Could you check a few things on this model? Use its own coordinates, in mm. A direction names the side the tool comes from. Round coordinates to 2 decimals unless told otherwise and drop trailing zeros. Write each loop counter-clockwise with the first axis right and the second up, starting at its lowest first coordinate (ties: lowest second). Pieces come first, ordered by that corner, then holes. Notation, with made-up numbers: M 35,42.25 L 78,42.25 A21 ccw 78,62.25 Z; hole C -29.75,57 d8. An arc over 180 degrees is marked long. One line per item, written item: value. Start each with the question number.
(1) Which directions (+Z, -Z, +X, -X, +Y, -Y) give clear straight access to the entire face, cutting with the end or side of a thin tool? Please do faces 4 (the face through (10.175, -5, 10)), 5 (the face through (-0.222, 6.984, 21.479)), 6 (the face through (3.32, 20.29, 17.54)), 7 (the face through (-9.906, -5, 10)).
(2) If I drill on L1, parallel to X at y = -4.5, z = 14.5; L2, parallel to Z at x = -0.5, y = 13; L3, parallel to Z at x = -4, y = 18.5, over which ranges is the centre line in solid material (lowest first)?
(3) I want a section at A-A on z = 1.5. Please give me the cut outline in (x, y), and give its area (3 significant figures).
(4) Thinking about a two-plate mould opening in Y: for faces 1 (the face through (14.93, 20.13, 9.86)), 2 (the face through (1.735, -1.567, 17.535)), 3 (the face through (15.17, 5.05, 9.86)), which applies, released by +Y, released by -Y, zero draft, split by the parting line, or undercut?
(5) I want a section at B-B on y = -3. Please give me the cut outline in (x, z), and give its area (3 significant figures).
(6) I want a section at C-C on x = -7. Please give me the cut outline in (y, z).
(7) I want a section at D-D on y = 22.5. Please give me the cut outline in (x, z), and give its area (3 significant figures).
(8) I'm going to push flat-ended pins straight in: pin 1 Ø6 at (x, y) = (-1, -1) entering from +Z; pin 2 Ø8 at (y, z) = (-5, 8) entering from +X; pin 3 Ø3 at (x, z) = (-14, 14) entering from +Y. Where does each tip first touch, or does it pass through?
```python
from build123d import *

# Parameters (mm, degrees)
PAD_DEPTH       = 20
POCKET_DEPTH    = 5
POCKET001_DEPTH = 5
PAD001_DEPTH    = 3


with BuildPart() as part:
    # Sketch → Pad (new body)
    with BuildSketch(Plane.XY):
        Polygon((-10.101072, 30.032787), (9.979783, 30.032787), (20.020205, 9.951933), (10.174738, 0), (10.174738, -9.836479), (-9.906112, -9.836479), (-9.906112, 0), (-20.141495, 9.854452), align=None)
    extrude(amount=PAD_DEPTH)

    # Sketch001 (on Face10 of Pad) → Pocket (cut)
    with BuildSketch(Plane.XY.offset(20)):
        Polygon((-6.373003, -1.744858), (-6.373003, -9.245775), (-5.063322, -9.126713), (-4.825196, -1.625796), align=None)
        Polygon((-3.158328, -1.506734), (-3.158328, -9.483899), (-1.253332, -9.364837), (-1.015209, -1.506734), align=None)
        Polygon((0.889791, -1.506734), (0.770723, -8.888589), (2.437592, -8.888589), (2.556656, -1.625796), align=None)
        Polygon((4.342592, -1.268609), (4.104469, -8.769526), (6.128524, -8.769526), (6.485711, -1.506734), align=None)
    extrude(amount=-POCKET_DEPTH, mode=Mode.SUBTRACT)

    # Sketch002 (on Face5 of Pocket) → Pocket001 (cut)
    with BuildSketch(Plane.XY.offset(20)):
        Polygon((-6.165723, 23.872267), (-9.380401, 17.56197), (-3.18917, 17.323847), align=None)
        Polygon((4.788002, 23.634144), (1.811443, 16.847597), (8.478922, 16.847597), align=None)
    extrude(amount=-POCKET001_DEPTH, mode=Mode.SUBTRACT)

    # Sketch004 (on Face5 of Pocket001) → Pad001 (join)
    with BuildSketch(Plane.XY.offset(20)):
        Polygon((0, 13.475349), (-3.27434, 6.807868), (2.916898, 7.165055), align=None)
    extrude(amount=PAD001_DEPTH)


solid = part.part
```
Found:
1. face 4: +Z, -Z, +X, -Y
1. face 5: +Z, +X, -Y
1. face 6: +Z
1. face 7: +Z, -Z, -X, -Y
2. L1: x = -9.91 to 10.17
2. L2: z = 0 to 20
2. L3: z = 0 to 15
3. outline: M -20.14,9.85 L -9.91,0 L -9.91,-9.84 L 10.17,-9.84 L 10.17,0 L 20.02,9.95 L 9.98,30.03 L -10.1,30.03 Z
3. area: 1,100 mm²
4. face 1: released by +Y
4. face 2: undercut
4. face 3: released by -Y
5. outline: M -9.91,0 L 10.17,0 L 10.17,20 L 6.41,20 L 6.41,15 L 4.29,15 L 4.29,20 L 2.53,20 L 2.53,15 L 0.87,15 L 0.87,20 L -1.06,20 L -1.06,15 L -3.16,15 L -3.16,20 L -4.87,20 L -4.87,15 L -6.37,15 L -6.37,20 L -9.91,20 Z
5. area: 365 mm²
6. outline: M -9.84,0 L 30.03,0 L 30.03,20 L 22.23,20 L 22.23,15 L 17.47,15 L 17.47,20 L -9.84,20 Z
7. outline: M -13.85,0 L 13.75,0 L 13.75,20 L 5.4,20 L 5.4,15 L 4.29,15 L 4.29,20 L -5.54,20 L -5.54,15 L -6.86,15 L -6.86,20 L -13.85,20 Z
7. area: 540 mm²
8. pin 1: stops at z = 20
8. pin 2: stops at x = 10.17
8. pin 3: stops at y = 25.21
